from build123d import *

# Parameters (mm, degrees)
SKETCH1_W               = 34.925
SKETCH1_H               = 38.1
BOSS_EXTRUDE1_DEPTH     = 3.175
SKETCH2_W               = 34.925
SKETCH2_H               = 9.525
BOSS_EXTRUDE2_DEPTH     = 24.3713
CUT_EXTRUDE1_START      = -16.4338
SKETCH3_R               = 11.1125
CUT_EXTRUDE1_DEPTH      = 25.3713
FILLET1_R               = 6.35
FILLET2_R               = 2.54
SKETCH4_R               = 4.9022
CUT_EXTRUDE2_DEPTH      = 4.175
F_3_8_CLEARANCE_HOLE1_D = 10.0838
F_6_CLEARANCE_HOLE1_D   = 4.3053
HOLE1_AT_2_COUNT        = 2
HOLE1_AT_2_PITCH        = 25.4
HOLE1_AT_3_COUNT        = 2
HOLE1_AT_3_PITCH        = 28.575
HOLE1_AT_4_COUNT        = 2
HOLE1_AT_4_PITCH        = 38.232062788
CUT_EXTRUDE3_REACH      = 29.546
SKETCH11_R              = 1.5875


with BuildPart() as part:
    # Sketch1 → Boss-Extrude1 (new body)
    with BuildSketch(Plane.XY):
        with Locations((-9.525, 0)):
            Rectangle(SKETCH1_W, SKETCH1_H)
    extrude(amount=BOSS_EXTRUDE1_DEPTH)

    # Sketch2 → Boss-Extrude2 (add)
    with BuildSketch(Plane.XY.offset(3.175)):
        with Locations((-9.525, 14.2875)):
            Rectangle(SKETCH2_W, SKETCH2_H)
    boss_extrude2 = extrude(amount=BOSS_EXTRUDE2_DEPTH)

    # Sketch3 → Cut-Extrude1 (cut)
    with BuildSketch(Plane.XY.offset(19.6088).offset(CUT_EXTRUDE1_START)):
        Circle(SKETCH3_R)
        with Locations((-19.05, 0)):
            Circle(SKETCH3_R)
    cut_extrude1 = extrude(amount=CUT_EXTRUDE1_DEPTH, mode=Mode.SUBTRACT)

    # Mirror1: Boss-Extrude2, Cut-Extrude1 across plane
    add(boss_extrude2.mirror(Plane.ZX))
    add(cut_extrude1.mirror(Plane.ZX), mode=Mode.SUBTRACT)

    # Fillet1
    fillet1_edges = [part.edges().sort_by_distance(p)[0] for p in [
        (7.9375, 19.05, 13.77315),
        (-26.9875, 19.05, 13.77315),
        (5.72381265, 9.525, 15.36065),
        (-5.72381265, 9.525, 15.36065),
        (-13.32618735, 9.525, 15.36065),
        (-24.77381265, 9.525, 15.36065),
        (7.9375, -19.05, 13.77315),
        (-26.9875, -19.05, 13.77315),
        (5.72381265, -9.525, 15.36065),
        (-5.72381265, -9.525, 15.36065),
        (-13.32618735, -9.525, 15.36065),
        (-24.77381265, -9.525, 15.36065),
    ]]
    fillet(fillet1_edges, radius=FILLET1_R)

    # Fillet2
    fillet2_edges = [part.edges().sort_by_distance(p)[0] for p in [
        (7.606169458, 9.525, 3.175),
        (5.921014367, 9.670996527, 3.175),
        (0, 11.1125, 3.175),
        (-5.921014367, 9.670996527, 3.175),
        (-9.525, 9.525, 3.175),
        (-13.128985633, 9.670996527, 3.175),
        (-19.05, 11.1125, 3.175),
        (-24.971014367, 9.670996527, 3.175),
        (-26.656169458, 9.525, 3.175),
        (7.606169458, -9.525, 3.175),
        (5.921014367, -9.670996527, 3.175),
        (0, -11.1125, 3.175),
        (-5.921014367, -9.670996527, 3.175),
        (-9.525, -9.525, 3.175),
        (-13.128985633, -9.670996527, 3.175),
        (-19.05, -11.1125, 3.175),
        (-24.971014367, -9.670996527, 3.175),
        (-26.656169458, -9.525, 3.175),
    ]]
    fillet(fillet2_edges, radius=FILLET2_R)

    # Sketch4 → Cut-Extrude2 (cut, through all)
    with BuildSketch(Plane.XY.offset(3.175)):
        with Locations((-19.05, 0)):
            Circle(SKETCH4_R)
    extrude(amount=-CUT_EXTRUDE2_DEPTH, mode=Mode.SUBTRACT)

    # 3/8 Clearance Hole1 (through all)
    with Locations(Plane.XY.offset(3.175)):
        with Locations((0, 0)):
            Hole(F_3_8_CLEARANCE_HOLE1_D / 2)

    # #6 Clearance Hole1 (through all)
    with Locations(Plane(origin=(0, 0, 0), x_dir=(-1, 0, 0), z_dir=(0, 0, -1))):
        with Locations((-3.175, 14.2875), (22.225, 14.2875), (22.225, -14.2875), (-3.175, -14.2875)):
            Hole(F_6_CLEARANCE_HOLE1_D / 2)

    # Sketch9 → Hole1 (revolve, cut)
    with BuildSketch(Plane(origin=(-22.225, 14.2875, 27.5463), x_dir=(0, -1, 0), z_dir=(1, 0, 0))):
        Polygon((0, 0), (0, 3.81), (2.5273, 3.81), (2.6543, 0), align=None)
    hole1 = revolve(axis=Axis((-22.225, 14.2875, -82.4537), (0, 0, 1)), mode=Mode.SUBTRACT)

    # Hole1 at 2: Hole1 ×2
    with Locations(*[(i * HOLE1_AT_2_PITCH, 0, 0) for i in range(1, HOLE1_AT_2_COUNT)]):
        add(hole1, mode=Mode.SUBTRACT)

    # Hole1 at 3: Hole1 ×2
    with Locations(*[(0, -i * HOLE1_AT_3_PITCH, 0) for i in range(1, HOLE1_AT_3_COUNT)]):
        add(hole1, mode=Mode.SUBTRACT)

    # Hole1 at 4: Hole1 ×2
    with Locations(*[Vector(0.664363839, -0.747409319, 0) * (i * HOLE1_AT_4_PITCH) for i in range(1, HOLE1_AT_4_COUNT)]):
        add(hole1, mode=Mode.SUBTRACT)

    # Sketch11 → Cut-Extrude3 (cut, up to next)
    with BuildSketch(Plane(origin=(0, 0, 0), x_dir=(-1, 0, 0), z_dir=(0, 0, -1)), mode=Mode.PRIVATE) as cut_extrude3_sk1:
        with Locations((23.8252, -8.270889016)):
            Circle(SKETCH11_R)
    cut_extrude3_tool1 = extrude(cut_extrude3_sk1.sketch, amount=-CUT_EXTRUDE3_REACH, mode=Mode.PRIVATE) & part.part
    add(cut_extrude3_tool1.solids().sort_by_distance((-23.8252, -8.270889, 0))[0], mode=Mode.SUBTRACT)

    # Sketch12 → Hole2 (revolve, cut)
    with BuildSketch(Plane(origin=(-22.225, 14.2875, 0), x_dir=(0, 1, 0), z_dir=(1, 0, 0))):
        Polygon((0, 0), (0, 3.81), (2.5273, 3.81), (2.6543, 0), align=None)
    revolve(axis=Axis((-22.225, 14.2875, 110), (0, 0, -1)), mode=Mode.SUBTRACT)


solid = part.part
Verification items for the finished model (mm, model axes). A direction names the side the tool comes from. Round coordinates to 2 decimals unless told otherwise and drop trailing zeros. Loops run counter-clockwise (first coordinate to the right, second up) from the corner with the lowest first, then second, coordinate; pieces in that order, holes last. Notation, with made-up numbers: (-3, 68.25) - (11, 68.25) arc R18 ccw to (11, 100.25) - close; hole circle Ø8 at (-14.75, -4). An arc over 180 degrees is marked (long way). Answer in a Markdown table with one row per item. Add a question column.
Q1. Gauge pin test, flat ends, axial feed: pin 1 (10 mm diameter, centred on x = -9.5, y = -4, fed in from +Z); pin 2 (5 mm diameter, centred on x = -20, y = -1.5, fed in from +Z); pin 3 (0.5 mm diameter, centred on x = 7.5, z = 18.5, fed in from -Y); pin 4 (8.5 mm diameter, centred on x = -10.5, y = -1, fed in from +Z) (3 decimals). Record the tip position at first contact, or that the pin passes through.
Q2. Section check A-A on y = 0. Enter the section's corners in (x, z) (1 decimal).
Q3. Release check for a two-part mould opening along Y. For faces 1 (the face through (6.127, -17.14, 13.966)), 2 (the face through (-10, -14, 27.546)), 3 (the face through (0.66, 5, 1.57)) record: pulls with the +Y half, pulls with the -Y half, needs draft (parallel to the pull), parting line crosses it, or undercut.
Q4. Material ranges on line 1 (Y direction, x = -7, z = 21.25); line 2 (Y direction, x = 4, z = 26.25); line 3 (Y direction, x = -19, z = 7.5), recorded low to high.
Q5. Section check C-C on z = 22.75. State how many separate pieces and enclosed holes the cut face has, plus the area to 3 significant figures.
Q6. Tool access check on faces 4 (the face through (-9.49, 8.76, 3.9)), 5 (the face through (5.902, 9.675, 16.478)), 6 (the face through (-14.374, 1.472, 1.61)). Record the directions out of +Z, -Z, +X, -X, +Y, -Y that give a thin tool (end or side, any length) a straight path to the whole face; none if there is none.
Found:
| question | item | result |
|---|---|---|
| 1 | pin 1 | stops at z = 4.17 |
| 1 | pin 2 | passes through |
| 1 | pin 3 | stops at y = -15.57 |
| 1 | pin 4 | stops at z = 3.175 |
| 2 | outline | (-27, 0) - (-24, 0) - (-24, 3.2) - (-27, 3.2) - close; (-14.1, 0) - (-5, 0) - (-5, 3.2) - (-14.1, 3.2) - close; (5, 0) - (7.9, 0) - (7.9, 3.2) - (5, 3.2) - close |
| 3 | face 1 | pulls with the -Y half |
| 3 | face 2 | needs draft |
| 3 | face 3 | undercut |
| 4 | line 1 | y = -19.05 to -9.53, 9.53 to 19.05 |
| 4 | line 2 | y = -18.57 to -16.76, -11.81 to -10.37, 10.37 to 11.81, 16.76 to 18.57 |
| 4 | line 3 | y = -19.05 to -11.11, 11.11 to 19.05 |
| 5 | separate pieces | 2 |
| 5 | enclosed holes | 4 |
| 5 | area | 522 mm² |
| 6 | face 4 | +Z, +X, -X |
| 6 | face 5 | +Z |
| 6 | face 6 | +Z, -Z |
